Here's how the part is built. I have some questions about the finished solid (model axes, mm). A direction names the side the tool comes from. Give positions to 0.01 mm unless a question says otherwise; leave off trailing zeros. Use one line per item in the form item = value.
Solid Edge part; units mm, degrees
sketch "Sketch1" plane through (0, 0, 0) normal (0, 0, 1) x (1, 0, 0)
  line L0 (0, 52.6414) -> (0.1414, 52.5)
  line L1 (0.1414, 52.5) -> (20.8586, 52.5)
  line L2 (20.8586, 52.5) -> (21, 52.6414)
  line L3 (21, 52.6414) -> (21, 67.5)
  arc A0 (21, 67.5) -> (18.5, 70) centre (18.5, 67.5) ccw
  line L4 (18.5, 70) -> (6, 70)
  arc A1 (6, 70) -> (4, 68) centre (6, 68) ccw
  line L5 (4, 68) -> (4, 58)
  arc A2 (4, 58) -> (2, 56) centre (2, 58) cw
  arc A3 (2, 56) -> (0, 54) centre (2, 54) ccw
  line L6 (0, 54) -> (0, 52.6414)
revolve "RevolvedProtrusion1" add sketch "Sketch1" angle 360 about axis through (50, 0, 0) along (-1, 0, 0)
sketch "Sketch2" plane through (21, 0, 0) normal (1, 0, 0) x (0, 1, 0)
  circle A0 centre (0, 0) radius 92.75
  line L0 (6, 69.7424) -> (6, 64.7424)
  line L1 (6, 64.7424) -> (-6, 64.7424)
  line L2 (-6, 64.7424) -> (-6, 69.7424)
  arc A1 (-6, 69.7424) -> (-69.7424, 6) centre (0, 0) ccw
  line L3 (-69.7424, 6) -> (-64.7424, 6)
  line L4 (-64.7424, 6) -> (-64.7424, -6)
  line L5 (-64.7424, -6) -> (-69.7424, -6)
  arc A2 (-69.7424, -6) -> (-6, -69.7424) centre (0, 0) ccw
  line L6 (-6, -69.7424) -> (-6, -64.7424)
  line L7 (-6, -64.7424) -> (6, -64.7424)
  line L8 (6, -64.7424) -> (6, -69.7424)
  arc A3 (6, -69.7424) -> (69.7424, -6) centre (0, 0) ccw
  line L9 (69.7424, -6) -> (64.7424, -6)
  line L10 (64.7424, -6) -> (64.7424, 6)
  line L11 (64.7424, 6) -> (69.7424, 6)
  arc A4 (69.7424, 6) -> (6, 69.7424) centre (0, 0) ccw
extrude "ExtrudedCutout_1" cut sketch "Sketch2" against normal blind 21
sketch "Sketch3" plane through (0, 40.2167, 40.2167) normal (0, 0.7071, 0.7071) x (1, 0, 0)
  circle A0 centre (12.5, 0) radius 5.1
extrude "ExtrudedCutout_2" cut sketch "Sketch3" along normal blind 22.75
sketch "Sketch4" plane through (0, 40.2167, 40.2167) normal (0, 0.7071, 0.7071) x (1, 0, 0)
  circle A0 centre (12.5, 0) radius 5.1
  line L0 (10.715, 1.0306) -> (10.715, -1.0306)
  line L1 (10.715, -1.0306) -> (12.5, -2.0611)
  line L2 (12.5, -2.0611) -> (14.285, -1.0306)
  line L3 (14.285, -1.0306) -> (14.285, 1.0306)
  line L4 (14.285, 1.0306) -> (12.5, 2.0611)
  line L5 (12.5, 2.0611) -> (10.715, 1.0306)
extrude "ExtrudedProtrusion_1" add sketch "Sketch4" along normal blind 13.125
(1) For P1, Ø1, axis at x = 14.5, y = -42.5, coming from the +Z side; P2, Ø3, axis at x = 14, z = 10, coming from the -Y side; P3, Ø1.5, axis at x = 15.5, z = 54, coming from the -Y side; P4, Ø9.5, axis at x = 15.5, y = -2.5, coming from the -Z side, each with a flat end and sliding along its axis, tell me the tip position at first contact or that it passes through.
Geometry says:
P1 = 56
P2 = -69.48
P3 = -45.44
P4 = -69.74
(2) For faces 1 (the flat face through (11.6, 43.7, 45.88)), 2 (the flat face through (13, 67, 6)), 3 (the flat face through (13, -67, -6)), 4 (the flat face through (13, 0, 64.742)), which set-ups out of +Z, -Z, +X, -X, +Y, -Y let a thin tool reach every point of the face, with its end or its side?
Geometry says:
face_1 = none
face_2 = +X, -X, +Y
face_3 = +X, -X, -Y
face_4 = +Z, +X, -X
(3) If I drill on probe 1 along Z at (x, y) = (7.25, 0); probe 2 along X at (y, z) = (-22, -56.5), over which ranges is the centre line in solid material (lowest first)?
Geometry says:
probe_1 = -64.74 to -52.5, 52.5 to 64.74
probe_2 = 4 to 21
(4) Thinking about a two-plate mould opening in Y: for faces 5 (the flat face through (13, -6, 67)), 6 (the flat face through (13, 64.742, 0)), 7 (the flat face through (0, 12, 52)), which applies, pulls with the +Y half, pulls with the -Y half, needs draft (parallel to the pull), parting line crosses it, or undercut?
Geometry says:
face_5 = undercut
face_6 = pulls with the +Y half
face_7 = needs draft
